The listing builds one solid part. Answer for the finished solid, in the listing's coordinates (mm). A direction names the side the tool comes from. Give positions to 0.01 mm unless a question says otherwise; leave off trailing zeros. Write each loop counter-clockwise with the first axis right and the second up, starting at its lowest first coordinate (ties: lowest second). Pieces come first, ordered by that corner, then holes. Notation, with made-up numbers: M 81,81 L 87,81 A17 ccw 87,112 Z; hole C 63.5,30 d10. An arc over 180 degrees is marked long. Answer as a JSON object with one key per item and string values.
```python
from build123d import *

# Parameters (mm, degrees)
BOSS_EXTRUDE1_DEPTH           = 10
CBORE_FOR_M3_SHCS1_AT_2_COUNT = 2
CBORE_FOR_M3_SHCS1_AT_2_PITCH = 20
CBORE_FOR_M3_SHCS1_AT_3_COUNT = 2
CBORE_FOR_M3_SHCS1_AT_3_PITCH = 28.284271247
CBORE_FOR_M3_SHCS1_AT_4_COUNT = 2
CBORE_FOR_M3_SHCS1_AT_4_PITCH = 20
CHAMFER1_SIZE                 = 0.4


with BuildPart() as part:
    # Sketch3 → Boss-Extrude1 (new body)
    with BuildSketch(Plane(origin=(0, 0, 0), x_dir=(1, 0, 0), z_dir=(0, 1, 0))):
        with BuildLine():
            Line((-14.85, -10), (-14.85, 10))
            ThreePointArc((-14.85, 10), (-13.429467889, 13.429467889), (-10, 14.85))
            Line((-10, 14.85), (10, 14.85))
            ThreePointArc((10, 14.85), (13.429467889, 13.429467889), (14.85, 10))
            Line((14.85, 10), (14.85, -10))
            ThreePointArc((14.85, -10), (13.429467889, -13.429467889), (10, -14.85))
            Line((10, -14.85), (-10, -14.85))
            ThreePointArc((-10, -14.85), (-13.429467889, -13.429467889), (-14.85, -10))
        make_face()
        Polygon((-6.15, 3.550704156), (-6.15, -3.550704156), (0, -7.101408311), (6.15, -3.550704156), (6.15, 3.550704156), (0, 7.101408311), align=None, mode=Mode.SUBTRACT)
    extrude(amount=BOSS_EXTRUDE1_DEPTH)

    # Sketch5 → CBORE for M3 SHCS1 (revolve, cut)
    with BuildSketch(Plane(origin=(-10, 10, -10), x_dir=(0, 0, 1), z_dir=(1, 0, 0))):
        Polygon((0, 0), (0, 10), (2.1, 10), (1.7, 9.6), (1.7, 3.4), (2.1, 3), (3.25, 3), (3.25, 0.4), (3.65, 0), align=None)
    cbore_for_m3_shcs1 = revolve(axis=Axis((-10, 16.35, -10), (0, -1, 0)), mode=Mode.SUBTRACT)

    # CBORE for M3 SHCS1 at 2: CBORE for M3 SHCS1 ×2
    with Locations(*[(i * CBORE_FOR_M3_SHCS1_AT_2_PITCH, 0, 0) for i in range(1, CBORE_FOR_M3_SHCS1_AT_2_COUNT)]):
        add(cbore_for_m3_shcs1, mode=Mode.SUBTRACT)

    # CBORE for M3 SHCS1 at 3: CBORE for M3 SHCS1 ×2
    with Locations(*[Vector(0.7071067811865476, 0, 0.7071067811865476) * (i * CBORE_FOR_M3_SHCS1_AT_3_PITCH) for i in range(1, CBORE_FOR_M3_SHCS1_AT_3_COUNT)]):
        add(cbore_for_m3_shcs1, mode=Mode.SUBTRACT)

    # CBORE for M3 SHCS1 at 4: CBORE for M3 SHCS1 ×2
    with Locations(*[(0, 0, i * CBORE_FOR_M3_SHCS1_AT_4_PITCH) for i in range(1, CBORE_FOR_M3_SHCS1_AT_4_COUNT)]):
        add(cbore_for_m3_shcs1, mode=Mode.SUBTRACT)

    # Chamfer1
    chamfer1_edges = [part.edges().sort_by_distance(p)[0] for p in [
        (14.85, 0, 0),
        (13.429467889, 0, 13.429467889),
        (0, 0, 14.85),
        (-13.429467889, 0, 13.429467889),
        (13.429467889, 10, 13.429467889),
        (14.85, 10, 0),
        (13.429467889, 10, -13.429467889),
        (0, 10, -14.85),
        (-3.075, 0, -5.326056233),
        (-6.15, 0, 0),
        (-3.075, 0, 5.326056233),
        (3.075, 0, 5.326056233),
        (6.15, 0, 0),
        (3.075, 0, -5.326056233),
        (-3.075, 10, -5.326056233),
        (-6.15, 10, 0),
        (-13.429467889, 10, -13.429467889),
        (-3.075, 10, 5.326056233),
        (3.075, 10, 5.326056233),
        (6.15, 10, 0),
        (3.075, 10, -5.326056233),
        (-14.85, 10, 0),
        (-13.429467889, 10, 13.429467889),
        (-14.85, 0, 0),
        (0, 10, 14.85),
        (-13.429467889, 0, -13.429467889),
        (0, 0, -14.85),
        (13.429467889, 0, -13.429467889),
    ]]
    chamfer(chamfer1_edges, length=CHAMFER1_SIZE)


solid = part.part
```
1. Consider line 1 along X through (y, z) = (8.75, -10); line 2 along X through (y, z) = (3.5, -10). Determine where each line is inside the solid, lowest interval first.
Verdict:
{"line 1": "x = -14.85 to -13.25, -6.75 to 6.75, 13.25 to 14.85", "line 2": "x = -14.85 to -11.7, -8.3 to 8.3, 11.7 to 14.85"}
2. A cutting plane is placed at C-C, the plane x = 3.5. Give the vertices of the cut face in (y, z).
Verdict:
{"outline": "M 0,-14.45 L 0.4,-14.85 L 9.6,-14.85 L 10,-14.45 L 10,-5.54 L 9.6,-5.08 L 0.4,-5.08 L 0,-5.54 Z; M 0,5.54 L 0.4,5.08 L 9.6,5.08 L 10,5.54 L 10,14.45 L 9.6,14.85 L 0.4,14.85 L 0,14.45 Z"}
3. A cutting plane is placed at B-B, the plane y = 8.75. Give the vertices of the cut face in (x, z), plus the area to 3 significant figures.
Verdict:
{"outline": "M -14.85,-10 A4.85 ccw -10,-14.85 L 10,-14.85 A4.85 ccw 14.85,-10 L 14.85,10 A4.85 ccw 10,14.85 L -10,14.85 A4.85 ccw -14.85,10 Z; hole C -10,-10 d6.5; hole C -10,10 d6.5; hole M -6.15,-3.55 L 0,-7.1 L 6.15,-3.55 L 6.15,3.55 L 0,7.1 L -6.15,3.55 Z; hole C 10,-10 d6.5; hole C 10,10 d6.5", "area": "598 mm2"}
4. A cutting plane is placed at D-D, the plane x = -9.25. Count the separate pieces of the cut face and the enclosed holes in it, plus the area to 3 significant figures.
Verdict:
{"separate pieces": "3", "enclosed holes": "0", "area": "215 mm2"}
5. A cutting plane is placed at A-A, the plane z = 0.5. Give the vertices of the cut face in (x, y).
Verdict:
{"outline": "M -14.85,0.4 L -14.45,0 L -6.55,0 L -6.15,0.4 L -6.15,9.6 L -6.55,10 L -14.45,10 L -14.85,9.6 Z; M 6.15,0.4 L 6.55,0 L 14.45,0 L 14.85,0.4 L 14.85,9.6 L 14.45,10 L 6.55,10 L 6.15,9.6 Z"}
6. The mould has two halves that part along Z. Classify faces 5 (the flat face through (7, 0, 0)), 6 (the flat face through (3.128, 0.203, 5.523)), 7 (the conical face through (-13.26, 0.11, -13.19)): released by +Z, released by -Z, zero draft, split by the parting line, or undercut.
Verdict:
{"face 5": "zero draft", "face 6": "undercut", "face 7": "released by -Z"}
7. Flat-ended cylindrical pins translate along their axes: pin 1 (5 mm diameter, centred on x = -10, z = -10, fed in from +Y); pin 2 (4 mm diameter, centred on x = 10, z = 10, fed in from +Y); pin 3 (3 mm diameter, centred on x = 9, z = -11.5, fed in from +Y). Find the tip coordinate at first contact, or state that the pin passes through.
Verdict:
{"pin 1": "stops at y = 7", "pin 2": "stops at y = 6.9", "pin 3": "stops at y = 9.65"}
8. For faces 1 (the flat face through (-3.219, 0.203, 5.47)), 2 (the flat face through (7, 10, 0)), 3 (the flat face through (6.15, 5, 0)), 4 (the cylindrical face through (-12.197, 8.318, 7.605)), determine the directions among +Z, -Z, +X, -X, +Y, -Y from which every point of the face is accessible in a straight line to the end or side of a thin tool.
Verdict:
{"face 1": "-Y", "face 2": "+Z, -Z, +X, -X, +Y", "face 3": "+Y, -Y", "face 4": "+Y"}
